```python
from build123d import *

# Parameters (mm, degrees)
SKETCH1_R           = 1.25
BOSS_EXTRUDE1_DEPTH = 16
SKETCH1_3_R         = 2.25
SKETCH1_3_R_2       = 1.25
BOSS_EXTRUDE2_DEPTH = 2.6
CUT_EXTRUDE1_DEPTH  = 1.4
FILLET1_R           = 0.2


with BuildPart() as part:
    # Sketch1 → Boss-Extrude1 (new body)
    with BuildSketch(Plane.XY):
        Circle(SKETCH1_R)
    extrude(amount=BOSS_EXTRUDE1_DEPTH)

    # Sketch1_3 → Boss-Extrude2 (add)
    with BuildSketch(Plane.XY):
        Circle(SKETCH1_3_R)
        Circle(SKETCH1_3_R_2, mode=Mode.SUBTRACT)
        Circle(SKETCH1_3_R_2)
    extrude(amount=-BOSS_EXTRUDE2_DEPTH)

    # Sketch2 → Cut-Extrude1 (cut)
    with BuildSketch(Plane(origin=(0, 0, -2.6), x_dir=(-1, 0, 0), z_dir=(0, 0, -1))):
        Polygon((0, 1.154700538), (-1, 0.577350269), (-1, -0.577350269), (0, -1.154700538), (1, -0.577350269), (1, 0.577350269), align=None)
    extrude(amount=-CUT_EXTRUDE1_DEPTH, mode=Mode.SUBTRACT)

    # Fillet1
    fillet1_edges = [part.edges().sort_by_distance(p)[0] for p in [
        (-1.25, 0, 16),
        (-2.25, 0, -2.6),
        (-2.25, 0, 0),
    ]]
    fillet(fillet1_edges, radius=FILLET1_R)


solid = part.part
```
Build history of the part. All positions in model axes, mm. A direction names the side the tool comes from. Round coordinates to 2 decimals unless told otherwise and drop trailing zeros. Write each loop counter-clockwise with the first axis right and the second up, starting at its lowest first coordinate (ties: lowest second). Pieces come first, ordered by that corner, then holes.
1) 3-axis set-ups, long thin cutter, end or side, ignore diameter. For faces 1 (the flat face through (-1, 0, -2)), 2 (the flat face through (1, -1, -2.6)): which of +Z, -Z, +X, -X, +Y, -Y reach the whole face in a straight line?
2) Band-saw the part on A-A, the plane y = 0. List the corners of the cut face in (x, z), and give its area (3 significant figures).
3) Band-saw the part on B-B, the plane z = 4. List the corners of the cut face in (x, y).
4) Drill centre lines: probe 1 along Z at (x, y) = (-1.2, -0.45); probe 2 along Y at (x, z) = (-0.75, 3.75); probe 3 along Z at (x, y) = (0.3, 0.75). Where is each one in solid material? Low to high.
5) Mould opens along Y. For faces 3 (the flat face through (0.51, -0.86, -1.91)), 4 (the flat face through (-1, -1, 0)), 5 (the cylindrical face through (-0.27, -1.22, 7.79)) say: +Y half, -Y half, draft (parallel to the pull), parting line (faces both ways), or undercut.
6) Pin check, flat tips, straight feed: pin 1 (1 mm diameter, centred on x = 1, z = 10.5, fed in from -Y); pin 2 (1.5 mm diameter, centred on x = -1.5, z = 1.5, fed in from +Y); pin 3 (1 mm diameter, centred on x = 0, z = 2.5, fed in from +Y). Stop position of each tip, or through.
Ans:
1. face 1: -Z
1. face 2: -Z, +X, -X, +Y, -Y
2. outline: (-2.25, -2.4) arc R0.2 ccw to (-2.05, -2.6) - (-1, -2.6) - (-1, -1.2) - (1, -1.2) - (1, -2.6) - (2.05, -2.6) arc R0.2 ccw to (2.25, -2.4) - (2.25, -0.2) arc R0.2 ccw to (2.05, 0) - (1.25, 0) - (1.25, 15.8) arc R0.2 ccw to (1.05, 16) - (-1.05, 16) arc R0.2 ccw to (-1.25, 15.8) - (-1.25, 0) - (-2.05, 0) arc R0.2 ccw to (-2.25, -0.2) - close
2. area: 48.8 mm2
3. outline: circle Ø2.5 at (0, 0)
4. probe 1: z = -2.6 to 0
4. probe 2: y = -1 to 1
4. probe 3: z = -1.2 to 16
5. face 3: undercut
5. face 4: draft
5. face 5: parting line
6. pin 1: stops at y = -1.15
6. pin 2: stops at y = 1
6. pin 3: stops at y = 1.25
